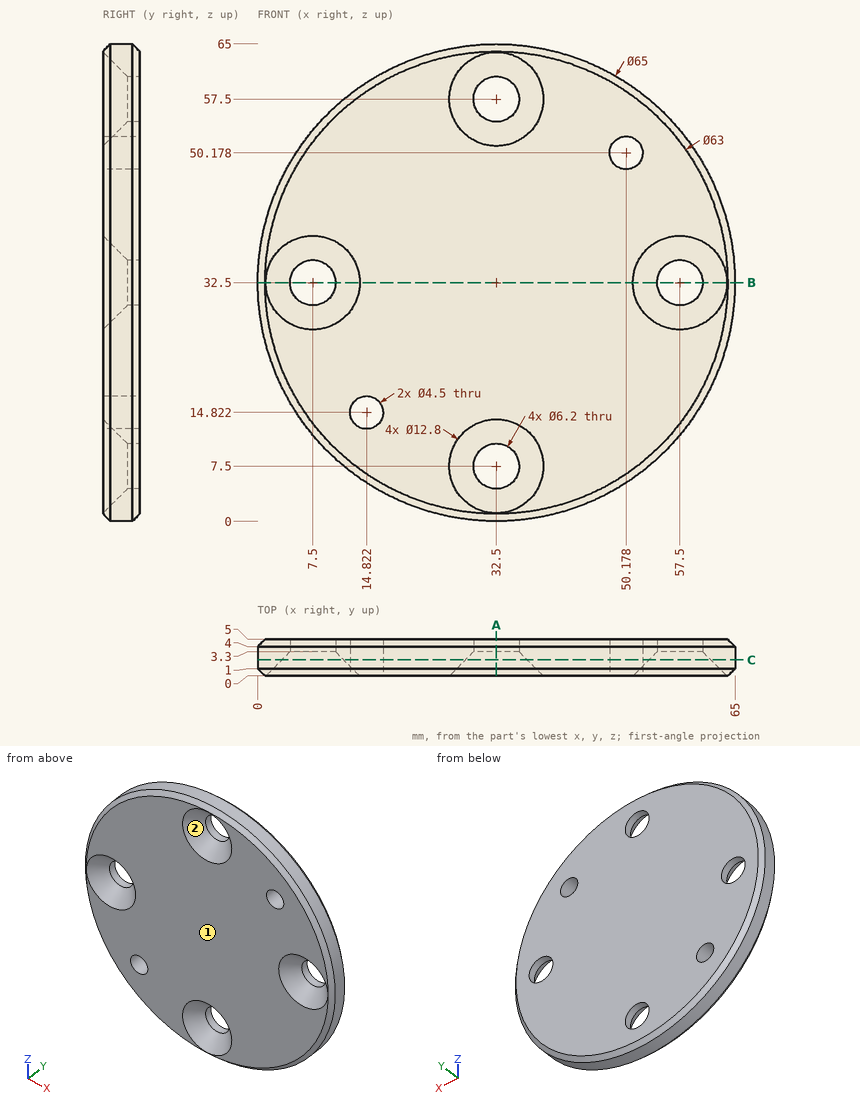
Verification items for this drawing (mm, ordinates from the low corner). Coordinates: 2 decimals unless noted, no trailing zeros. Write each loop counter-clockwise with the first axis right and the second up, starting at its lowest first coordinate (ties: lowest second). Pieces come first, ordered by that corner, then holes. Notation, with made-up numbers: (18.5, 79) -> (43.5, 79) arc R16 cw to (43.5, 84) -> close; hole circle Ø2 at (-14, 13). An arc over 180 degrees is marked (long way). One line per item, written item: value. Start each with the question number.
Q1. Cross-section at A-A on x = 32.5. Enter the section's corners in (y, z).
Q2. Mould release check, pull along X, two halves, no side actions. Record for the marked faces 1 and 2: pulls with the +X half, pulls with the -X half, needs draft (parallel to the pull), parting line crosses it, or undercut.
Q3. Thickness scan on L1, parallel to X at y = 3.85, z = 32.5; L2, parallel to Z at x = 38, y = 0.2 (1 decimal); L3, parallel to X at y = 4.05, z = 32.5. Record the ranges inside material, lowest first. Write a range as from..to.
Q4. Cross-section at B-B on z = 32.5. Enter the section's corners in (x, y).
Q5. Cross-section at C-C on y = 2.2. Enter the section's corners in (x, z).
Q6. Go/stop test with flat-tipped pins: P1, Ø1.5, axis at x = 45.5, y = 3.5, coming from the +Z side; P2, Ø5.5, axis at x = 57.5, z = 32.5, coming from the -Y side; P3, Ø10, axis at x = 32.5, z = 57.5, coming from the -Y side; P4, Ø1, axis at x = 35, z = 55.5, coming from the -Y side. Record where each tip stops, or that it passes through.
Checked values:
1. outline: (0, 1) -> (1, 0) -> (4, 0) -> (5, 1) -> (5, 4.4) -> (3.3, 4.4) -> (0, 1.1) -> close; (0, 13.9) -> (3.3, 10.6) -> (5, 10.6) -> (5, 54.4) -> (3.3, 54.4) -> (0, 51.1) -> close; (0, 63.9) -> (3.3, 60.6) -> (5, 60.6) -> (5, 64) -> (4, 65) -> (1, 65) -> (0, 64) -> close
2. face 1: needs draft
2. face 2: undercut
3. L1: x = 0..4.4, 10.6..54.4, 60.6..65
3. L2: z = 1.3..4.6, 10.4..54.6, 60.4..63.7
3. L3: x = 0.05..4.4, 10.6..54.4, 60.6..64.95
4. outline: (0, 1) -> (1, 0) -> (1.1, 0) -> (4.4, 3.3) -> (4.4, 5) -> (1, 5) -> (0, 4) -> close; (10.6, 3.3) -> (13.9, 0) -> (51.1, 0) -> (54.4, 3.3) -> (54.4, 5) -> (10.6, 5) -> close; (60.6, 3.3) -> (63.9, 0) -> (64, 0) -> (65, 1) -> (65, 4) -> (64, 5) -> (60.6, 5) -> close
5. outline: circle Ø65 at (32.5, 32.5); hole circle Ø8.4 at (7.5, 32.5); hole circle Ø4.5 at (14.82, 14.82); hole circle Ø8.4 at (32.5, 7.5); hole circle Ø8.4 at (32.5, 57.5); hole circle Ø4.5 at (50.18, 50.18); hole circle Ø8.4 at (57.5, 32.5)
6. P1: stops at z = 62.6
6. P2: passes through
6. P3: stops at y = 1.4
6. P4: stops at y = 2.7
